Design review of the part built by this model. Coordinates are the model's own, in mm. A direction names the side the tool comes from. Give positions to 0.01 mm unless a question says otherwise; leave off trailing zeros. Write each loop counter-clockwise with the first axis right and the second up, starting at its lowest first coordinate (ties: lowest second). Pieces come first, ordered by that corner, then holes.
```python
from build123d import *

# Parameters (mm, degrees)
SKETCH1_R           = 32
SKETCH1_R_2         = 12.5
BOSS_EXTRUDE1_DEPTH = 15
SKETCH2_R           = 10
CUT_EXTRUDE1_DEPTH  = 56.689497751
CIRPATTERN1_COUNT   = 3
SKETCH4_R           = 3
CUT_EXTRUDE3_DEPTH  = 11
CIRPATTERN2_COUNT   = 3
CHAMFER2_SIZE       = 2


with BuildPart() as part:
    # Sketch1 → Boss-Extrude1 (new, symmetric)
    with BuildSketch(Plane.XY):
        Circle(SKETCH1_R)
        Circle(SKETCH1_R_2, mode=Mode.SUBTRACT)
    extrude(amount=BOSS_EXTRUDE1_DEPTH, both=True)

    # Sketch2 → Cut-Extrude1 (cut, through all)
    with BuildSketch(Plane(origin=(0, -9.819536819, -3.123093004), x_dir=(1, 0, 0), z_dir=(0, 0.9510565162951555, 0.3090169943749417))):
        with Locations(Location((0, -7.935834199, 0), (0, 0, 270))):
            Circle(SKETCH2_R)
    cut_extrude1 = extrude(amount=-CUT_EXTRUDE1_DEPTH, mode=Mode.SUBTRACT)

    # CirPattern1: Cut-Extrude1 ×3 about axis
    cirpattern1_axis = Axis((0, 0, 0), (0, 0, 1))
    for i in range(1, CIRPATTERN1_COUNT):
        add(cut_extrude1.rotate(cirpattern1_axis, i * 360 / CIRPATTERN1_COUNT), mode=Mode.SUBTRACT)

    # Sketch4 → Cut-Extrude3 (cut)
    with BuildSketch(Plane.XY.offset(-15)):
        with Locations(Location((0, -22, 0), (0, 0, 180))):
            Circle(SKETCH4_R)
    cut_extrude3 = extrude(amount=CUT_EXTRUDE3_DEPTH, mode=Mode.SUBTRACT)

    # CirPattern2: Cut-Extrude3 ×3 about axis
    cirpattern2_axis = Axis((0, 0, 0), (0, 0, 1))
    for i in range(1, CIRPATTERN2_COUNT):
        add(cut_extrude3.rotate(cirpattern2_axis, i * 360 / CIRPATTERN2_COUNT), mode=Mode.SUBTRACT)

    # Chamfer2
    chamfer2_edges = [part.edges().sort_by_distance(p)[0] for p in [
        (-32, 0, -15),
    ]]
    chamfer(chamfer2_edges, length=CHAMFER2_SIZE)


solid = part.part
```
(1) Clearance check with flat-ended pins moving along their axes: P1, Ø5.5, axis at x = 19.05, y = 11, coming from the -Z side; P2, Ø3, axis at x = 8, z = 5.5, coming from the -Y side; P3, Ø3, axis at y = 18, z = -4, coming from the +X side; P4, Ø8, axis at x = -1, y = -19.5, coming from the -Z side. State where each tip first meets the part, or that it passes through.
Resolved:
P1: stops at z = 10.89
P2: stops at y = -31.31
P3: stops at x = 16.33
P4: stops at z = -15
(2) Tool access review of faces 4 (the face through (11.547, -4.788, -0.21)), 5 (the face through (-16.055, 10.868, -11.685)), 6 (the face through (-11.59, 6.53, 7.59)): name each direction out of +Z, -Z, +X, -X, +Y, -Y from which nothing blocks a thin tool from reaching the whole face with its end or side.
Resolved:
face 4: +Z, -Z
face 5: -Z
face 6: none
(3) Consider section B-B, the plane y = 10.5. Give the number of separate pieces and of enclosed holes in the cut face, then the cut area to 3 significant figures.
Resolved:
separate pieces: 6
enclosed holes: 0
area: 466 mm2
(4) Consider section A-A, the plane x = 0. Give the boundary of the cut face in (y, z), then the cut area to 3 significant figures.
Resolved:
outline: (-32, -13) - (-30, -15) - (-25, -15) - (-25, -10.23) - (-32, -12.5) - close; (-32, 8.53) - (-15.36, 13.93) - (-12.5, 5.13) - (-12.5, 15) - (-32, 15) - close; (-19, -15) - (-12.5, -15) - (-12.5, -6.16) - (-19, -8.28) - close; (12.5, -15) - (30, -15) - (32, -13) - (32, 15) - (12.5, 15) - close
area: 735 mm2
(5) To check wall thickness, follow L1, parallel to X at y = 11, z = -11; L2, parallel to Y at x = -10.5, z = 10; L3, parallel to X at y = 0.5, z = 4. State the ranges of each line that lie inside material, in increasing order.
Resolved:
L1: x = -30.05 to -22.05, -16.05 to -5.94, 5.94 to 16.05, 22.05 to 30.05
L2: y = -30.23 to -6.78, 6.78 to 9.98, 14.74 to 30.23
L3: x = -32 to -20.67, -13.72 to -12.49, 12.49 to 13.72, 20.67 to 32
(6) Mouldability with a two-part tool opening along Y and no side actions: class faces 1 (the face through (11.45, 6.77, 7.59)), 2 (the face through (0, -13, -15)), 3 (the face through (14.766, -28.39, 1.196)) as pulls with the +Y half, pulls with the -Y half, needs draft (parallel to the pull), parting line crosses it, or undercut.
Resolved:
face 1: undercut
face 2: needs draft
face 3: parting line crosses it
